Autodesk Inventor part; units mm, degrees
ref_plane "YZ Plane" through (0, 0, 0) normal (1, 0, 0) x (0, 1, 0)
ref_plane "XZ Plane" through (0, 0, 0) normal (0, 1, 0) x (-1, 0, 0)
ref_plane "XY Plane" through (0, 0, 0) normal (0, 0, 1) x (1, 0, 0)
sketch "Skizze1" plane through (0, 0, 0) normal (0, 0, 1) x (1, 0, 0)
  line L0 (-2.5, -2.5) -> (2.5, -2.5)
  line L1 (2.5, -2.5) -> (2.5, 2.5)
  line L2 (2.5, 2.5) -> (-2.5, 2.5)
  line L3 (-2.5, 2.5) -> (-2.5, -2.5)
  line L4 (-2.5, -2.5) -> (2.5, 2.5) construction
  line L5 (2.5, -2.5) -> (-2.5, 2.5) construction
  point P0 (0, 0)
  dimension "d0" = 5
  dimension "d1" = 5
extrude "Extrusion1" add sketch "Skizze1" against normal blind 40
sketch "Skizze3" plane through (-2.5, -2.5, 0) normal (-1, 0, 0) x (0, 0, 1)
  line L0 (0, 5) -> (-40, 5)
  line L1 (-40, 0) -> (-40, 5)
  line L2 (0, 0) -> (-40, 0)
  line L3 (-35, 5) -> (-40, 5)
  line L4 (-40, 5) -> (-40, 0)
  line L5 (-40, 0) -> (-35, 0)
  line L6 (-35, 0) -> (-35, 5)
  line L7 (-35, 5) -> (-40, 0) construction
  line L8 (-40, 5) -> (-35, 0) construction
  point P0 (0, 2.5)
  point P1 (-37.5, 2.5)
  point P2 (-40, 2.5)
  point P3 (-35, 0)
  point P4 (-35, 5)
  dimension "d14" = 5
  dimension "d15" = 5
sketch "Skizze4" plane through (2.5, -2.5, 0) normal (1, 0, 0) x (0, 0, -1)
  line L0 (0, 0) -> (40, 0)
  line L1 (40, 5) -> (40, 0)
  line L2 (0, 5) -> (40, 5)
  line L3 (35, 5) -> (40, 5)
  line L4 (40, 5) -> (40, 0)
  line L5 (40, 0) -> (35, 0)
  line L6 (35, 0) -> (35, 5)
  line L7 (35, 5) -> (40, 0) construction
  line L8 (40, 5) -> (35, 0) construction
  point P0 (0, 2.5)
  point P1 (37.5, 2.5)
  point P2 (40, 2.5)
  point P3 (35, 5)
  point P4 (35, 0)
  dimension "d16" = 5
  dimension "d17" = 5
extrude "Extrusion2" add sketch "Skizze4" along normal blind 10
extrude "Extrusion3" add sketch "Skizze3" along normal blind 10
sketch "Skizze5" plane through (0, 0, -40) normal (0, 0, -1) x (-1, 0, 0)
  line L0 (12.5, -2.5) -> (-12.5, -2.5)
  line L1 (12.5, 2.5) -> (12.5, -2.5)
  line L2 (-12.5, 2.5) -> (12.5, 2.5)
  line L3 (-12.5, -2.5) -> (-12.5, 2.5)
  line L4 (12.5, -2.5) -> (7.5, -2.5)
  line L5 (7.5, -2.5) -> (7.5, 2.5)
  line L6 (7.5, 2.5) -> (12.5, 2.5)
  line L7 (12.5, 2.5) -> (12.5, -2.5)
  line L8 (12.5, -2.5) -> (7.5, 2.5) construction
  line L9 (7.5, -2.5) -> (12.5, 2.5) construction
  line L10 (-7.5, 2.5) -> (-12.5, 2.5)
  line L11 (-12.5, 2.5) -> (-12.5, -2.5)
  line L12 (-12.5, -2.5) -> (-7.5, -2.5)
  line L13 (-7.5, -2.5) -> (-7.5, 2.5)
  line L14 (-7.5, 2.5) -> (-12.5, -2.5) construction
  line L15 (-12.5, 2.5) -> (-7.5, -2.5) construction
  point P0 (0, 0)
  point P1 (10, 0)
  point P2 (-10, 0)
  point P3 (12.5, 0)
  point P4 (-12.5, 0)
  point P5 (7.5, 2.5)
  dimension "d22" = 5
  dimension "d23" = 5
  dimension "d24" = 5
  dimension "d25" = 5
extrude "Extrusion4" add sketch "Skizze5" along normal blind 40 contours L0 L5 L2 L1 | L0 L3 L2 L13
sketch "Skizze6" plane through (-12.5, -2.5, 0) normal (-1, 0, 0) x (0, 0, 1)
  line L0 (-80, 0) -> (-80, 5)
  line L1 (-35, 0) -> (-80, 0)
  point P0 (0, 2.5)
  point P1 (-70, 2.5)
  point P2 (-80, 2.5)
  dimension "d35" = 10
  dimension "d36" = 2.5
hole "Bohrung2" at (-12.5, 0, -70) direction (1, 0, 0) diameter 3 end through all
sketch "Skizze7" plane through (12.5, -2.5, 0) normal (1, 0, 0) x (0, 0, -1)
  circle A0 centre (70, 2.5) radius 1.5
  line L0 (35, 0) -> (80, 0)
  line L1 (80, 5) -> (80, 0)
  line L2 (35, 5) -> (80, 5)
  line L3 (35, 5) -> (35, 0)
  point P0 (0, 2.5)
sketch "Skizze8" plane through (-12.5, -2.5, 0) normal (-1, 0, 0) x (0, 0, 1)
  line L0 (-35, 0) -> (-80, 0)
  line L1 (-35, 0) -> (-35, 5)
  point P0 (0, 2.5)
  point P1 (-37.5, 2.5)
  dimension "d44" = 2.5
  dimension "d45" = 2.5
hole "Bohrung1" at (-12.5, 0, -37.5) direction (1, 0, 0) diameter 4 end through all
fillet "Rundung1" radius 2 10 edges at (-7.5, 0, -80) (7.5, 0, -80) (-12.5, 0, -80) (12.5, 0, -80) (2.5, 0, 0) (-2.5, 0, 0) (0, 2.5, 0) (0, -2.5, 0) (-2.5, 0, -35) (2.5, 0, -35)
properties part number "Hebel"
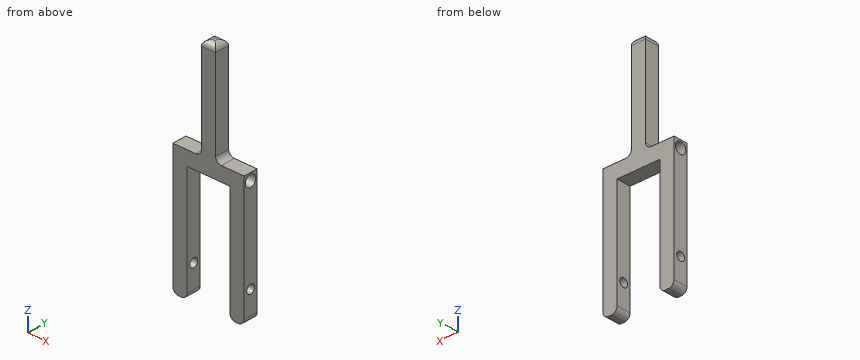
Can you work these out from the model? Positions are in its coordinate system, mm. Give positions to 0.01 mm unless a question says otherwise; leave off trailing zeros. Loops run counter-clockwise (first coordinate to the right, second up) from the corner with the lowest first, then second, coordinate; pieces in that order, holes last. Notation, with made-up numbers: (42.25, 81.25) - (91.25, 81.25) arc R21 cw to (91.25, 98.25) - close; hole circle Ø3 at (44, -15.75). An arc over 180 degrees is marked (long way). Return JSON: item names as keys, results as strings.
1. I want a section at C-C on z = -55. Please give me the cut outline in (x, y).
Output values:
{"outline": "(-12.5, -2.5) - (-7.5, -2.5) - (-7.5, 2.5) - (-12.5, 2.5) - close; (7.5, -2.5) - (12.5, -2.5) - (12.5, 2.5) - (7.5, 2.5) - close"}
2. If I drill on line 1 (Z direction, x = 9.6, y = 0); line 2 (X direction, y = -1.95, z = -53.5); line 3 (Y direction, x = -9.4, z = -70), over which ranges is the centre line in solid material (lowest first)?
Output values:
{"line 1": "z = -80 to -71.5, -68.5 to -39.5, -35.5 to -35", "line 2": "x = -12.5 to -7.5, 7.5 to 12.5", "line 3": "y = -2.5 to -1.5, 1.5 to 2.5"}
3. I'm going to push flat-ended pins straight in: pin 1 Ø3 at (y, z) = (1.5, -15.5) entering from -X; pin 2 Ø1.5 at (x, y) = (9.5, 0.5) entering from +Z; pin 3 Ø2.5 at (y, z) = (0, -70) entering from -X. Where does each tip first touch, or does it pass through?
Output values:
{"pin 1": "stops at x = -2.5", "pin 2": "stops at z = -35", "pin 3": "passes through"}
4. I want a section at A-A on z = -37.5. Please give me the cut outline in (x, y).
Output values:
{"outline": "(-12.5, -2.5) - (12.5, -2.5) - (12.5, -2) - (-12.5, -2) - close; (-12.5, 2) - (12.5, 2) - (12.5, 2.5) - (-12.5, 2.5) - close"}
5. I want a section at B-B on z = -70. Please give me the cut outline in (x, y), and give its area (3 significant figures).
Output values:
{"outline": "(-12.5, -2.5) - (-7.5, -2.5) - (-7.5, -1.5) - (-12.5, -1.5) - close; (-12.5, 1.5) - (-7.5, 1.5) - (-7.5, 2.5) - (-12.5, 2.5) - close; (7.5, -2.5) - (12.5, -2.5) - (12.5, -1.5) - (7.5, -1.5) - close; (7.5, 1.5) - (12.5, 1.5) - (12.5, 2.5) - (7.5, 2.5) - close", "area": "20.0 mm²"}
